```python
from build123d import *
from OCP.BRepFilletAPI import BRepFilletAPI_MakeChamfer

# Parameters (mm, degrees)
ESQUISSE1_W             = 35
ESQUISSE1_H             = 28
ESQUISSE1_W_2           = 77
ESQUISSE1_H_2           = 52
BOSS_EXTRU_1_DEPTH      = 1.6
ENL_V_MAT_EXTRU_1_REACH = 94.928
ESQUISSE2_R             = 1.5
BOSS_EXTRU_2_DEPTH      = 2
BOSS_EXTRU_2_DEPTH_BACK = 13
ESQUISSE3_R             = 1.016
CHANFREIN1_SIZE         = 2
CHANFREIN1_SIZE_2       = 0.6


with BuildPart() as part:
    # Esquisse1 → Boss.-Extru.1 (new body)
    with BuildSketch(Plane(origin=(0, 0, 0), x_dir=(1, 0, 0), z_dir=(0, 1, 0))):
        with Locations((-17.5, 26)):
            Rectangle(ESQUISSE1_W, ESQUISSE1_H)
        with Locations((38.5, 26)):
            Rectangle(ESQUISSE1_W_2, ESQUISSE1_H_2)
    extrude(amount=BOSS_EXTRU_1_DEPTH)

    # Esquisse2 → Enlèv. mat.-Extru.1 (cut, up to next)
    with BuildSketch(Plane(origin=(0, 1.6, 0), x_dir=(1, 0, 0), z_dir=(0, 1, 0)), mode=Mode.PRIVATE) as enl_v_mat_extru_1_sk1:
        with Locations(Location((-31, 36, 0), (0, 0, 270))):
            Circle(ESQUISSE2_R)
    enl_v_mat_extru_1_tool1 = extrude(enl_v_mat_extru_1_sk1.sketch, amount=-ENL_V_MAT_EXTRU_1_REACH, mode=Mode.PRIVATE) & part.part
    # Esquisse2 → Enlèv. mat.-Extru.1 (cut, up to next)
    with BuildSketch(Plane(origin=(0, 1.6, 0), x_dir=(1, 0, 0), z_dir=(0, 1, 0)), mode=Mode.PRIVATE) as enl_v_mat_extru_1_sk2:
        with Locations(Location((-31, 16, 0), (0, 0, 270))):
            Circle(ESQUISSE2_R)
    enl_v_mat_extru_1_tool2 = extrude(enl_v_mat_extru_1_sk2.sketch, amount=-ENL_V_MAT_EXTRU_1_REACH, mode=Mode.PRIVATE) & part.part
    # Esquisse2 → Enlèv. mat.-Extru.1 (cut, up to next)
    with BuildSketch(Plane(origin=(0, 1.6, 0), x_dir=(1, 0, 0), z_dir=(0, 1, 0)), mode=Mode.PRIVATE) as enl_v_mat_extru_1_sk3:
        with Locations(Location((4, 4, 0), (0, 0, 270))):
            Circle(ESQUISSE2_R)
    enl_v_mat_extru_1_tool3 = extrude(enl_v_mat_extru_1_sk3.sketch, amount=-ENL_V_MAT_EXTRU_1_REACH, mode=Mode.PRIVATE) & part.part
    # Esquisse2 → Enlèv. mat.-Extru.1 (cut, up to next)
    with BuildSketch(Plane(origin=(0, 1.6, 0), x_dir=(1, 0, 0), z_dir=(0, 1, 0)), mode=Mode.PRIVATE) as enl_v_mat_extru_1_sk4:
        with Locations(Location((4, 48, 0), (0, 0, 270))):
            Circle(ESQUISSE2_R)
    enl_v_mat_extru_1_tool4 = extrude(enl_v_mat_extru_1_sk4.sketch, amount=-ENL_V_MAT_EXTRU_1_REACH, mode=Mode.PRIVATE) & part.part
    # Esquisse2 → Enlèv. mat.-Extru.1 (cut, up to next)
    with BuildSketch(Plane(origin=(0, 1.6, 0), x_dir=(1, 0, 0), z_dir=(0, 1, 0)), mode=Mode.PRIVATE) as enl_v_mat_extru_1_sk5:
        with Locations(Location((73, 48, 0), (0, 0, 270))):
            Circle(ESQUISSE2_R)
    enl_v_mat_extru_1_tool5 = extrude(enl_v_mat_extru_1_sk5.sketch, amount=-ENL_V_MAT_EXTRU_1_REACH, mode=Mode.PRIVATE) & part.part
    # Esquisse2 → Enlèv. mat.-Extru.1 (cut, up to next)
    with BuildSketch(Plane(origin=(0, 1.6, 0), x_dir=(1, 0, 0), z_dir=(0, 1, 0)), mode=Mode.PRIVATE) as enl_v_mat_extru_1_sk6:
        with Locations(Location((73, 4, 0), (0, 0, 270))):
            Circle(ESQUISSE2_R)
    enl_v_mat_extru_1_tool6 = extrude(enl_v_mat_extru_1_sk6.sketch, amount=-ENL_V_MAT_EXTRU_1_REACH, mode=Mode.PRIVATE) & part.part
    add(enl_v_mat_extru_1_tool1.solids().sort_by_distance((-31, 1.6, -36))[0], mode=Mode.SUBTRACT)
    add(enl_v_mat_extru_1_tool2.solids().sort_by_distance((-31, 1.6, -16))[0], mode=Mode.SUBTRACT)
    add(enl_v_mat_extru_1_tool3.solids().sort_by_distance((4, 1.6, -4))[0], mode=Mode.SUBTRACT)
    add(enl_v_mat_extru_1_tool4.solids().sort_by_distance((4, 1.6, -48))[0], mode=Mode.SUBTRACT)
    add(enl_v_mat_extru_1_tool5.solids().sort_by_distance((73, 1.6, -48))[0], mode=Mode.SUBTRACT)
    add(enl_v_mat_extru_1_tool6.solids().sort_by_distance((73, 1.6, -4))[0], mode=Mode.SUBTRACT)

    # Esquisse3 → Boss.-Extru.2 (add, two sides: drawn at the far end of the back side and taken through both)
    with BuildSketch(Plane(origin=(0, 1.6, 0), x_dir=(1, 0, 0), z_dir=(0, 1, 0)).offset(-BOSS_EXTRU_2_DEPTH_BACK)):
        with Locations(Location((-31, 31, 0), (0, 0, 270))):
            Circle(ESQUISSE3_R)
        with Locations(Location((-31, 28.46, 0), (0, 0, 270))):
            Circle(ESQUISSE3_R)
        with Locations(Location((-31, 25.92, 0), (0, 0, 270))):
            Circle(ESQUISSE3_R)
        with Locations(Location((-31, 23.38, 0), (0, 0, 270))):
            Circle(ESQUISSE3_R)
        with Locations(Location((-31, 20.84, 0), (0, 0, 270))):
            Circle(ESQUISSE3_R)
    extrude(amount=BOSS_EXTRU_2_DEPTH + BOSS_EXTRU_2_DEPTH_BACK)

    # Chanfrein1
    chanfrein1_edges_1 = [part.edges().sort_by_distance(p)[0] for p in [
        (-31, 3.6, -32.016),
    ]]
    chanfrein1_side_1 = [part.faces().sort_by_distance(p)[0] for p in [
        (-31, 3.588, -32.016),
    ]]
    chanfrein1_edges_2 = [part.edges().sort_by_distance(p)[0] for p in [
        (-31, 3.6, -29.476),
    ]]
    chanfrein1_side_2 = [part.faces().sort_by_distance(p)[0] for p in [
        (-31, 3.588, -29.476),
    ]]
    chanfrein1_edges_3 = [part.edges().sort_by_distance(p)[0] for p in [
        (-31, 3.6, -26.936),
    ]]
    chanfrein1_side_3 = [part.faces().sort_by_distance(p)[0] for p in [
        (-31, 3.588, -26.936),
    ]]
    chanfrein1_edges_4 = [part.edges().sort_by_distance(p)[0] for p in [
        (-31, 3.6, -24.396),
    ]]
    chanfrein1_side_4 = [part.faces().sort_by_distance(p)[0] for p in [
        (-31, 3.588, -24.396),
    ]]
    chanfrein1_edges_5 = [part.edges().sort_by_distance(p)[0] for p in [
        (-31, 3.6, -21.856),
    ]]
    chanfrein1_side_5 = [part.faces().sort_by_distance(p)[0] for p in [
        (-31, 3.588, -21.856),
    ]]
    chanfrein1 = BRepFilletAPI_MakeChamfer(part.part.solid().wrapped)
    for e in chanfrein1_edges_1:
        chanfrein1.Add(CHANFREIN1_SIZE - 0.0001, CHANFREIN1_SIZE_2 - 0.0001, e.wrapped, chanfrein1_side_1[0].wrapped)
    for e in chanfrein1_edges_2:
        chanfrein1.Add(CHANFREIN1_SIZE - 0.0001, CHANFREIN1_SIZE_2 - 0.0001, e.wrapped, chanfrein1_side_2[0].wrapped)
    for e in chanfrein1_edges_3:
        chanfrein1.Add(CHANFREIN1_SIZE - 0.0001, CHANFREIN1_SIZE_2 - 0.0001, e.wrapped, chanfrein1_side_3[0].wrapped)
    for e in chanfrein1_edges_4:
        chanfrein1.Add(CHANFREIN1_SIZE - 0.0001, CHANFREIN1_SIZE_2 - 0.0001, e.wrapped, chanfrein1_side_4[0].wrapped)
    for e in chanfrein1_edges_5:
        chanfrein1.Add(CHANFREIN1_SIZE - 0.0001, CHANFREIN1_SIZE_2 - 0.0001, e.wrapped, chanfrein1_side_5[0].wrapped)
    add(Compound.cast(chanfrein1.Shape()), mode=Mode.REPLACE)  # a hair under: the kernel refuses the full size


solid = part.part
```
CAD build for the part. Positions are in the model's coordinates, mm. A direction names the side the tool comes from. Give positions to 0.01 mm unless a question says otherwise; leave off trailing zeros. Loops run counter-clockwise (first coordinate to the right, second up) from the corner with the lowest first, then second, coordinate; pieces in that order, holes last. Notation, with made-up numbers: M 75.5,18.25 L 124.5,18.25 A6 cw 124.5,22.25 Z; hole C 9,26 d2. An arc over 180 degrees is marked long. Use one line per item in the form item = value.
Item 1: Flat gauge pins, fed straight in: pin 1 (0.8 mm diameter, centred on x = -21.5, y = 0.5, fed in from -Z); pin 2 (5 mm diameter, centred on x = 40.5, z = -44.5, fed in from +Y); pin 3 (1 mm diameter, centred on y = -7, z = -22, fed in from -X); pin 4 (3 mm diameter, centred on x = 17.5, y = 1, fed in from +Z). Where does each tip first touch, or does it go through?
Determined:
pin_1 = -40
pin_2 = 1.6
pin_3 = -31.77
pin_4 = 0
Item 2: Two-plate mould, pull along X, no slides. Class faces 3 (the face through (74.01, 0.81, -49.11)), 4 (the face through (-31.39, 2.84, -31.51)), 5 (the face through (33, 0, -26)): pulls with the +X half, pulls with the -X half, needs draft (parallel to the pull), parting line crosses it, or undercut.
Determined:
face_3 = undercut
face_4 = parting line crosses it
face_5 = needs draft
Item 3: Slice it at C-C (x = 73). List the corners of the cut face in (y, z).
Determined:
outline = M 0,-52 L 1.6,-52 L 1.6,-49.5 L 0,-49.5 Z; M 0,-46.5 L 1.6,-46.5 L 1.6,-5.5 L 0,-5.5 Z; M 0,-2.5 L 1.6,-2.5 L 1.6,0 L 0,0 Z
Item 4: Which spindle directions (+Z, -Z, +X, -X, +Y, -Y) get a long thin tool onto all of the face, cutting with end or side? Do faces 1 (the face through (74.265, 0.811, -3.194)), 2 (the face through (-30.143, -5.78, -25.374)). Say none if no direction does.
Determined:
face_1 = +Y, -Y
face_2 = -Y
Item 5: Slice it at A-A (z = -36). List the corners of the cut face in (x, y), plus the area to 3 significant figures.
Determined:
outline = M -35,0 L -32.5,0 L -32.5,1.6 L -35,1.6 Z; M -29.5,0 L 77,0 L 77,1.6 L -29.5,1.6 Z
area = 174 mm2
Item 6: Drill centre lines: probe 1 along X at (y, z) = (1.25, -4); probe 2 along X at (y, z) = (0.75, -16); probe 3 along Y at (x, z) = (21.5, -31). Where is each one in solid material? Low to high. Write a range as from..to.
Determined:
probe_1 = 0..2.5, 5.5..71.5, 74.5..77
probe_2 = -35..-32.5, -29.5..77
probe_3 = 0..1.6
Item 7: Slice it at D-D (y = -10.25). List the corners of the cut face in (x, z).
Determined:
outline = C -31,-31 d2.03; C -31,-28.46 d2.03; C -31,-25.92 d2.03; C -31,-23.38 d2.03; C -31,-20.84 d2.03
Item 8: Slice it at B-B (z = -48). List the corners of the cut face in (x, y).
Determined:
outline = M 0,0 L 2.5,0 L 2.5,1.6 L 0,1.6 Z; M 5.5,0 L 71.5,0 L 71.5,1.6 L 5.5,1.6 Z; M 74.5,0 L 77,0 L 77,1.6 L 74.5,1.6 Z
